```python
from build123d import *

# Parameters (mm, degrees)
BOSS_EXTRUDE1_DEPTH      = 38.1
FILLET1_START            = -39
FILLET1_DEPTH            = 78
FILLET1_START_2          = -38.1
FILLET1_2_DEPTH          = 76.2
M8_CLEARANCE_HOLE1_D     = 8.4
M8_CLEARANCE_HOLE1_DEPTH = 10.668
M8_CLEARANCE_HOLE1_TIP   = 2.5236146
M5_CLEARANCE_HOLE8_D     = 5.3
M5_CLEARANCE_HOLE8_DEPTH = 4.318
M5_CLEARANCE_HOLE9_D     = 5.3
M5_CLEARANCE_HOLE9_DEPTH = 4.318


with BuildPart() as part:
    # Sketch1 → Boss-Extrude1 (new, symmetric)
    with BuildSketch(Plane.XY):
        Polygon((-101.6, -100.710476364), (-69.85, -100.710476364), (-69.85, -49.910476364), (-101.6, -49.910476364), (-101.6, -54.228476364), (-74.168, -54.228476364), (-74.168, -96.392476364), (-101.6, -96.392476364), align=None)
    extrude(amount=BOSS_EXTRUDE1_DEPTH, both=True)

    # Fillet1: read off the stored shape, not the designer's step
    # Fillet1 outline → Fillet1 (cut)
    with BuildSketch(Plane.XY.offset(FILLET1_START)):
        with BuildLine():
            Line((-101.6, -54.228476364), (-97.282, -54.228476364))
            ThreePointArc((-97.282, -54.228476364), (-100.335287081, -52.963763446), (-101.6, -49.910476364))
            Line((-101.6, -49.910476364), (-101.6, -54.228476364))
        make_face()
        with BuildLine():
            ThreePointArc((-101.6, -100.710476364), (-100.335287081, -97.657189283), (-97.282, -96.392476364))
            Line((-97.282, -96.392476364), (-101.6, -96.392476364))
            Line((-101.6, -96.392476364), (-101.6, -100.710476364))
        make_face()
    extrude(amount=FILLET1_DEPTH, mode=Mode.SUBTRACT)

    # Fillet1 2 outline → Fillet1 2 (add)
    with BuildSketch(Plane.XY.offset(FILLET1_START_2)):
        with BuildLine():
            Line((-74.168, -96.392476364), (-74.168, -92.074476364))
            ThreePointArc((-74.168, -92.074476364), (-75.432712919, -95.127763446), (-78.486, -96.392476364))
            Line((-78.486, -96.392476364), (-74.168, -96.392476364))
        make_face()
        with BuildLine():
            Line((-74.168, -54.228476364), (-78.486, -54.228476364))
            ThreePointArc((-78.486, -54.228476364), (-75.432712919, -55.493189283), (-74.168, -58.546476364))
            Line((-74.168, -58.546476364), (-74.168, -54.228476364))
        make_face()
    extrude(amount=FILLET1_2_DEPTH)

    # M8 Clearance Hole1
    with Locations(Plane(origin=(-6.8, -43.560476364, 0), x_dir=(1, 0, 0), z_dir=(0, 1, 0))):
        with Locations((84.25, 0), (-84.25, 0)):
            Hole(M8_CLEARANCE_HOLE1_D / 2, depth=M8_CLEARANCE_HOLE1_DEPTH)
            with Locations((0, 0, -(M8_CLEARANCE_HOLE1_DEPTH + M8_CLEARANCE_HOLE1_TIP / 2))):  # 118° drill point
                Cone(0, M8_CLEARANCE_HOLE1_D / 2, M8_CLEARANCE_HOLE1_TIP, mode=Mode.SUBTRACT)

    # M5 Clearance Hole8
    with Locations(Plane(origin=(-6.8, -49.910476364, 0), x_dir=(-1, 0, 0), z_dir=(0, 1, 0))):
        with Locations((81.25, 25), (81.25, -25), (-81.25, -25), (-81.25, 25)):
            Hole(M5_CLEARANCE_HOLE8_D / 2, depth=M5_CLEARANCE_HOLE8_DEPTH)

    # M5 Clearance Hole9
    with Locations(Plane(origin=(-6.8, -100.710476364, 0), x_dir=(1, 0, 0), z_dir=(0, -1, 0))):
        with Locations((-81.25, -25), (-81.25, 25), (83.05, 25), (83.05, -25), (-84.25, 0), (84.25, 0)):
            Hole(M5_CLEARANCE_HOLE9_D / 2, depth=M5_CLEARANCE_HOLE9_DEPTH)


solid = part.part
```
Input: part model. Units: mm. Frame: model coordinates. A direction names the side the tool comes from. Give positions to 0.01 mm unless a question says otherwise; leave off trailing zeros. Loops run counter-clockwise (first coordinate to the right, second up) from the corner with the lowest first, then second, coordinate; pieces in that order, holes last. Notation, with made-up numbers: (14.25, 32) -> (42.25, 32) arc R12 ccw to (42.25, 47) -> close; hole circle Ø7 at (77, 20). An arc over 180 degrees is marked (long way). Use a Markdown table: item, result.
Q1. Section query A-A, the plane z = -25. Return the cut outline in (x, y).
Entries:
| item | result |
|---|---|
| outline | (-101.6, -100.71) -> (-90.7, -100.71) -> (-90.7, -96.39) -> (-97.28, -96.39) arc R4.32 ccw to start; (-101.6, -49.91) arc R4.32 ccw to (-97.28, -54.23) -> (-90.7, -54.23) -> (-90.7, -49.91) -> close; (-85.4, -100.71) -> (-69.85, -100.71) -> (-69.85, -49.91) -> (-85.4, -49.91) -> (-85.4, -54.23) -> (-78.49, -54.23) arc R4.32 cw to (-74.17, -58.55) -> (-74.17, -92.07) arc R4.32 cw to (-78.49, -96.39) -> (-85.4, -96.39) -> close |
Q2. Section query D-D, the plane y = -70.5. Return the cut outline in (x, z), plus the area to 3 significant figures.
Entries:
| item | result |
|---|---|
| outline | (-74.17, -38.1) -> (-69.85, -38.1) -> (-69.85, 38.1) -> (-74.17, 38.1) -> close |
| area | 329 mm² |
Q3. Ray query, probe 1 along Z at (x, y) = (-88.05, -98.3); probe 2 along Y at (x, z) = (-91, 11.5); probe 3 along Z at (x, y) = (-91, -53). Return the intervals inside material, ascending. Write a range as from..to.
Entries:
| item | result |
|---|---|
| probe 1 | z = -38.1..-27.65, -22.35..22.35, 27.65..38.1 |
| probe 2 | y = -100.71..-96.39, -54.23..-49.91 |
| probe 3 | z = -38.1..-4.2, 4.2..38.1 |
Q4. First-contact query: P1, Ø12, axis at y = -68.5, z = -10, coming from the -X side; P2, Ø3, axis at x = -88.05, z = 25, coming from the +Y side; P3, Ø7.5, axis at x = -91.05, z = 0, coming from the +Y side. Flat tips, straight axial feed; report the tip coordinate or a pass-through.
Entries:
| item | result |
|---|---|
| P1 | stops at x = -74.17 |
| P2 | passes through |
| P3 | stops at y = -96.39 |
Q5. Pull-direction query (Z, two-part tool) for faces 4 (the cylindrical face through (-90.5, -98.52, 23.99)), 5 (the flat face through (-86, -54.228, 1)), 6 (the flat face through (-74, -77, -38.1)), 7 (the cylindrical face through (-93.578, -98.521, 0.796)); classes: pulls with the +Z half, pulls with the -Z half, needs draft (parallel to the pull), parting line crosses it, or undercut.
Entries:
| item | result |
|---|---|
| face 4 | undercut |
| face 5 | needs draft |
| face 6 | pulls with the -Z half |
| face 7 | undercut |
Q6. Section query B-B, the plane x = -82. Return the cut outline in (y, z), plus the area to 3 significant figures.
Entries:
| item | result |
|---|---|
| outline | (-100.71, -38.1) -> (-96.39, -38.1) -> (-96.39, 38.1) -> (-100.71, 38.1) -> close; (-54.23, -38.1) -> (-49.91, -38.1) -> (-49.91, 38.1) -> (-54.23, 38.1) -> close |
| area | 658 mm² |
Q7. Access query for faces 1 (the flat face through (-74, -77, 38.1)), 2 (the cylindrical face through (-86.854, -52.1, -0.185)), 3 (the cylindrical face through (-75.399, -95.094, -0.533)). Directions: +Z, -Z, +X, -X, +Y, -Y. A direction counts if a zero-diameter tool reaches every point of the face in a straight line with its end or side. Return the directions, or none.
Entries:
| item | result |
|---|---|
| face 1 | +Z, +X, -X, +Y, -Y |
| face 2 | +Y |
| face 3 | +Z, -Z, -X |
Q8. Section query C-C, the plane z = 26.5. Return the cut outline in (x, y), plus the area to 3 significant figures.
Entries:
| item | result |
|---|---|
| outline | (-101.6, -100.71) -> (-90.23, -100.71) -> (-90.23, -96.39) -> (-97.28, -96.39) arc R4.32 ccw to start; (-101.6, -49.91) arc R4.32 ccw to (-97.28, -54.23) -> (-90.23, -54.23) -> (-90.23, -49.91) -> close; (-85.87, -100.71) -> (-69.85, -100.71) -> (-69.85, -49.91) -> (-85.87, -49.91) -> (-85.87, -54.23) -> (-78.49, -54.23) arc R4.32 cw to (-74.17, -58.55) -> (-74.17, -92.07) arc R4.32 cw to (-78.49, -96.39) -> (-85.87, -96.39) -> close |
| area | 419 mm² |
